```python
from build123d import *

# Parameters (mm, degrees)
F0_R     = 11.2
F1_DEPTH = 7


with BuildPart() as f1:
    # F0 (on Top) → F1 (new body)
    with BuildSketch(Plane.XY):
        with BuildLine():
            ThreePointArc((10.3281411328, 8.2200669548), (10.1972511679, 8.3717102549), (10.074000709, 8.5296254147))
            ThreePointArc((10.074000709, 8.5296254147), (7.4035330811, 10.9282980338), (4.1855750451, 12.5188242875))
            ThreePointArc((4.1855750451, 12.5188242875), (-0.3452490992, 13.1954841919), (-4.8344899154, 12.2828216326))
            ThreePointArc((-4.8344899154, 12.2828216326), (-7.7506695625, 10.6849015593), (-10.1749836281, 8.4089064788))
            ThreePointArc((-10.1749836281, 8.4089064788), (-4.468233214, -12.4207444199), (13.2, 0))
            ThreePointArc((13.2, 0), (12.4613695666, 4.3536500231), (10.3281411328, 8.2200669548))
        make_face()
        Circle(F0_R, mode=Mode.SUBTRACT)
        with BuildLine():
            ThreePointArc((10.3281411328, 8.2200669548), (10.2022450736, 8.3758101374), (10.074000709, 8.5296254147))
            ThreePointArc((10.074000709, 8.5296254147), (10.1972511679, 8.3717102549), (10.3281411328, 8.2200669548))
        make_face()
        with BuildLine():
            ThreePointArc((4.1855750451, 12.5188242875), (7.4035330811, 10.9282980338), (10.074000709, 8.5296254147))
            Line((10.074000709, 8.5296254147), (7.6865181327, 19.9412759393))
            Line((7.6865181327, 19.9412759393), (4.1855750451, 12.5188242875))
        make_face()
        with BuildLine():
            ThreePointArc((15.8676719554, 7.7748145738), (13.0097806042, 6.901037059), (10.3281411328, 8.2200669548))
            ThreePointArc((10.3281411328, 8.2200669548), (12.4613695666, 4.3536500231), (13.2, 0))
            ThreePointArc((13.2, 0), (-4.468233214, -12.4207444199), (-10.1749836281, 8.4089064788))
            ThreePointArc((-10.1749836281, 8.4089064788), (-15.9654138837, 8.2058267338), (-18.2521417737, 13.5294720531))
            Line((-18.2521417737, 13.5294720531), (-28.0488785159, 13.1921837517))
            ThreePointArc((-28.0488785159, 13.1921837517), (-18.4228655221, 9.4930316), (-14.3946892798, 0))
            ThreePointArc((-14.3946892798, 0), (-15.9784644263, -6.2692360104), (-20.3497377879, -11.034068963))
            ThreePointArc((-20.3497377879, -11.034068963), (-7.2156496997, -17.8748402529), (0, -30.8067705482))
            ThreePointArc((0, -30.8067705482), (8.1731824308, -18.8997973628), (20.7994515503, -11.8887881909))
            ThreePointArc((20.7994515503, -11.8887881909), (13.7315728101, -3.2112002777), (15.8676719554, 7.7748145738))
        make_face()
        with BuildLine():
            ThreePointArc((-10.1749836281, 8.4089064788), (-7.7506695625, 10.6849015593), (-4.8344899154, 12.2828216326))
            Line((-4.8344899154, 12.2828216326), (-7.4686547741, 19.3583834916))
            Line((-7.4686547741, 19.3583834916), (-10.1749836281, 8.4089064788))
        make_face()
        with BuildLine():
            ThreePointArc((16.9216233027, 9.0455875637), (16.4599264938, 8.356060205), (15.8676719554, 7.7748145738))
            ThreePointArc((15.8676719554, 7.7748145738), (13.7315728101, -3.2112002777), (20.7994515503, -11.8887881909))
            ThreePointArc((20.7994515503, -11.8887881909), (22.7350911295, -11.4067904706), (24.6973457089, -11.0482108434))
            ThreePointArc((24.6973457089, -11.0482108434), (19.2942274575, 8.5446451852), (37.735017377, 0))
            ThreePointArc((37.735017377, 0), (35.5470001475, -6.6501253029), (29.8378447798, -10.7019311877))
            ThreePointArc((29.8378447798, -10.7019311877), (31.8304630475, -10.7940985486), (33.8132592946, -11.0121385111))
            ThreePointArc((33.8132592946, -11.0121385111), (36.1041313286, -9.0924176202), (37.9043873019, -6.7065212675))
            ThreePointArc((37.9043873019, -6.7065212675), (38.4946332583, -2.9960688252), (39.7233684855, 0.5544321757))
            ThreePointArc((39.7233684855, 0.5544321757), (35.6651689499, 9.5331176566), (26.5196883397, 13.1999910993))
            ThreePointArc((26.5196883397, 13.1999910993), (21.2916554427, 12.1139240392), (16.9216233027, 9.0455875637))
        make_face()
        with BuildLine():
            ThreePointArc((16.9216233027, 9.0455875637), (16.3747607551, 8.4266948075), (15.8676719554, 7.7748145738))
            ThreePointArc((15.8676719554, 7.7748145738), (16.4599264938, 8.356060205), (16.9216233027, 9.0455875637))
        make_face()
        with BuildLine():
            ThreePointArc((16.7203744661, 13.1886111726), (17.3900464241, 11.1447410536), (16.9216233027, 9.0455875637))
            ThreePointArc((16.9216233027, 9.0455875637), (21.2916554427, 12.1139240392), (26.5196883397, 13.1999910993))
            Line((26.5196883397, 13.1999910993), (16.7203744661, 13.1886111726))
        make_face()
        with BuildLine():
            ThreePointArc((24.6973457089, -11.0482108434), (22.7350911295, -11.4067904706), (20.7994515503, -11.8887881909))
            ThreePointArc((20.7994515503, -11.8887881909), (27.4221988949, -13.1701521994), (33.8132592946, -11.0121385111))
            ThreePointArc((33.8132592946, -11.0121385111), (31.8304630475, -10.7940985486), (29.8378447798, -10.7019311877))
            ThreePointArc((29.8378447798, -10.7019311877), (27.2877774528, -11.1746745934), (24.6973457089, -11.0482108434))
        make_face()
        with BuildLine():
            Line((59.2723935843, 13.2380267605), (26.5196883397, 13.1999910993))
            ThreePointArc((26.5196883397, 13.1999910993), (35.6651689499, 9.5331176566), (39.7233684855, 0.5544321757))
            ThreePointArc((39.7233684855, 0.5544321757), (47.6248104741, 9.7831637012), (59.2723935843, 13.2380267605))
        make_face()
        with BuildLine():
            ThreePointArc((37.9043873019, -6.7065212675), (36.1041313286, -9.0924176202), (33.8132592946, -11.0121385111))
            Line((33.8132592946, -11.0121385111), (38.8711988926, -14.7407511249))
            ThreePointArc((38.8711988926, -14.7407511249), (38.0054073492, -10.769651182), (37.9043873019, -6.7065212675))
        make_face()
        with BuildLine():
            ThreePointArc((-14.3946892798, 0), (-18.4228655221, 9.4930316), (-28.0488785159, 13.1921837517))
            ThreePointArc((-28.0488785159, 13.1921837517), (-38.1058502056, 7.9847038763), (-40.4254078025, -3.1004293559))
            ThreePointArc((-40.4254078025, -3.1004293559), (-40.2568023788, -3.6563255049), (-40.103121039, -4.2165311485))
            ThreePointArc((-40.103121039, -4.2165311485), (-37.4932231177, -8.7326415168), (-33.3377120847, -11.8851878009))
            ThreePointArc((-33.3377120847, -11.8851878009), (-31.5807696858, -11.3708961265), (-29.791803972, -10.9823807542))
            ThreePointArc((-29.791803972, -10.9823807542), (-34.6951229091, 8.6616304629), (-16.3946892798, 0))
            ThreePointArc((-16.3946892798, 0), (-18.4872924031, -6.5188436191), (-23.9831396603, -10.6017314315))
            ThreePointArc((-23.9831396603, -10.6017314315), (-22.1587710386, -10.7534603081), (-20.3497377879, -11.034068963))
            ThreePointArc((-20.3497377879, -11.034068963), (-15.9784644263, -6.2692360104), (-14.3946892798, 0))
        make_face()
        with BuildLine():
            ThreePointArc((-40.4254078025, -3.1004293559), (-38.1058502056, 7.9847038763), (-28.0488785159, 13.1921837517))
            Line((-28.0488785159, 13.1921837517), (-61.8749952175, 12.02759663))
            ThreePointArc((-61.8749952175, 12.02759663), (-48.6070915858, 8.069385126), (-40.4254078025, -3.1004293559))
        make_face()
        with BuildLine():
            ThreePointArc((39.735017377, 0), (39.7321048328, 0.2772772683), (39.7233684855, 0.5544321757))
            ThreePointArc((39.7233684855, 0.5544321757), (38.4946332583, -2.9960688252), (37.9043873019, -6.7065212675))
            ThreePointArc((37.9043873019, -6.7065212675), (39.2691385286, -3.4759399442), (39.735017377, 0))
        make_face()
        with BuildLine():
            ThreePointArc((-33.3377120847, -11.8851878009), (-26.7315274964, -13.1717482414), (-20.3497377879, -11.034068963))
            ThreePointArc((-20.3497377879, -11.034068963), (-22.1587710386, -10.7534603081), (-23.9831396603, -10.6017314315))
            ThreePointArc((-23.9831396603, -10.6017314315), (-26.8623095848, -11.1760288109), (-29.791803972, -10.9823807542))
            ThreePointArc((-29.791803972, -10.9823807542), (-31.5807696858, -11.3708961265), (-33.3377120847, -11.8851878009))
        make_face()
        with BuildLine():
            ThreePointArc((-40.103121039, -4.2165311485), (-40.2568023788, -3.6563255049), (-40.4254078025, -3.1004293559))
            ThreePointArc((-40.4254078025, -3.1004293559), (-40.2765485699, -3.6620274365), (-40.103121039, -4.2165311485))
        make_face()
        with BuildLine():
            Line((-40.1510037482, -15.3303835541), (-33.3377120847, -11.8851878009))
            ThreePointArc((-33.3377120847, -11.8851878009), (-37.4932231177, -8.7326415168), (-40.103121039, -4.2165311485))
            ThreePointArc((-40.103121039, -4.2165311485), (-39.4042920046, -9.7765713214), (-40.1510037482, -15.3303835541))
        make_face()
    extrude(amount=F1_DEPTH)


solid = f1.part
```
Geometry check sheet. Reference: the model listing, model coordinates, mm. A direction names the side the tool comes from. Coordinates: 2 decimals unless noted, no trailing zeros. Loops run counter-clockwise (first coordinate to the right, second up) from the corner with the lowest first, then second, coordinate; pieces in that order, holes last. Notation, with made-up numbers: (-25.75, -29) - (-1.75, -29) arc R36 ccw to (-1.75, 7) - close; hole circle Ø11 at (5.25, 33). An arc over 180 degrees is marked (long way). One line per item, written item: value. Start each with the question number.
(1) Tool access check on faces 1 (the cylindrical face through (47.5, 9.7, 3.5)), 2 (the flat face through (-36.79, -13.63, 3.45)), 3 (the cylindrical face through (17.39, 11.18, 3.45)), 4 (the flat face through (5.96, 16.28, 3.45)). Record the directions out of +Z, -Z, +X, -X, +Y, -Y that give a thin tool (end or side, any length) a straight path to the whole face; none if there is none.
(2) Cross-section at B-B on x = 2. Enter the section's corners in (y, z).
(3) Depth check by flat-ended pin: P1, Ø4, axis at y = 1, z = 1, coming from the +X side; P2, Ø13.5, axis at x = 0, y = 0, coming from the -Z side; P3, Ø1, axis at x = -20.5, z = 2.5, coming from the +Y side; P4, Ø3, axis at y = -12.5, z = 3, coming from the -X side. Enter the tip coordinate at first touch or a pass-through.
(4) Cross-section at D-D on y = 5. Enter the section's corners in (x, z).
(5) Material ranges on line 1 (X direction, y = -13.5, z = 4.5); line 2 (X direction, y = -4.5, z = 0.75); line 3 (X direction, y = -8, z = 6), recorded low to high. Write a range as [from, to].
(6) Mould release check, pull along X, two halves, no side actions. Record for faces 5 (the flat face through (-8.803, 13.96, 3.451)), 6 (the cylindrical face through (-39.404, -9.698, 3.451)), 7 (the flat face through (-11, -5, 0)): released by +X, released by -X, zero draft, split by the parting line, or undercut.
(7) Cross-section at A-A on z = 4.5. Enter the section's corners in (x, y) (1 decimal), plus the area to 3 significant figures.
(8) Cross-section at C-C on y = -9.5. Enter the section's corners in (x, z).
Results below:
1. face 1: +Z, -Z, +X, -Y
1. face 2: +Z, -Z, -Y
1. face 3: +Z, -Z
1. face 4: +Z, -Z, +Y
2. outline: (-26.61, 0) - (-11.02, 0) - (-11.02, 7) - (-26.61, 7) - close; (11.02, 0) - (13.05, 0) - (13.05, 7) - (11.02, 7) - close
3. P1: stops at x = 41.01
3. P2: passes through
3. P3: stops at y = 13.47
3. P4: stops at x = -39.84
4. outline: (-45.12, 0) - (-37.62, 0) - (-37.62, 7) - (-45.12, 7) - close; (-17.57, 0) - (-10.02, 0) - (-10.02, 7) - (-17.57, 7) - close; (10.02, 0) - (16.51, 0) - (16.51, 7) - (10.02, 7) - close; (36.56, 0) - (42.4, 0) - (42.4, 7) - (36.56, 7) - close
5. line 1: x = [-39.74, -36.53], [-13.27, 16.39], [37.19, 38.52]
5. line 2: x = [-40.03, -37.85], [-17.34, -10.26], [10.26, 16.28], [36.79, 38.94]
5. line 3: x = [-39.47, -35.43], [-19.76, -7.84], [7.84, 18.7], [34.37, 37.85]
6. face 5: undercut
6. face 6: released by -X
6. face 7: zero draft
7. outline: (-61.9, 12) arc R21.7 cw to (-40.4, -3.1) arc R13.2 ccw to (-40.1, -4.2) arc R21.7 cw to (-40.2, -15.3) - (-33.3, -11.9) arc R13.2 ccw to (-20.3, -11) arc R25.8 cw to (0, -30.8) arc R31.5 cw to (20.8, -11.9) arc R13.2 ccw to (33.8, -11) - (38.9, -14.7) arc R21.4 cw to (37.9, -6.7) arc R13.2 ccw to (39.7, 0.6) arc R21.4 cw to (59.3, 13.2) - (16.7, 13.2) arc R4.1 cw to (16.9, 9) arc R13.2 ccw to (15.9, 7.8) arc R4.1 cw to (10.3, 8.2) arc R13.2 ccw to (10.1, 8.5) - (7.7, 19.9) - (4.2, 12.5) arc R13.2 ccw to (-4.8, 12.3) - (-7.5, 19.4) - (-10.2, 8.4) arc R5.1 cw to (-18.3, 13.5) - close; hole circle Ø22.4 at (-27.6, 0); hole circle Ø22.4 at (0, 0); hole circle Ø22.4 at (26.5, 0)
7. area: 1,180 mm2
8. outline: (-39.4, 0) - (-33.53, 0) - (-33.53, 7) - (-39.4, 7) - close; (-21.66, 0) - (-5.93, 0) - (-5.93, 7) - (-21.66, 7) - close; (5.93, 0) - (20.6, 0) - (20.6, 7) - (5.93, 7) - close; (32.47, 0) - (37.89, 0) - (37.89, 7) - (32.47, 7) - close
